Source: CAD feature listing. Evaluate the final solid. Frame: model axes, mm. Face numbers are marked on the shaded views. Coordinates: 2 decimals unless noted, no trailing zeros. Loops run counter-clockwise (first coordinate to the right, second up) from the corner with the lowest first, then second, coordinate; pieces in that order, holes last.
Item 1: Section query D-D, the plane z = -0.45. Return the cut outline in (x, y), then the cut area to 3 significant figures.
Item 2: Section query A-A, the plane x = 0. Return the cut outline in (y, z).
Item 3: Pin query (flat end, axial travel): pin 1 Ø6 at (x, y) = (2, -3.5) entering from +Z; pin 2 Ø5 at (x, y) = (0, 0) entering from -Z; pin 3 Ø1 at (y, z) = (-7.5, -0.5) entering from +X; pin 4 Ø2 at (x, z) = (7.5, 0.5) entering from -Y. Return the tip coordinate at first contact, or that it passes through.
Item 4: Section query C-C, the plane y = -5.5. Return the cut outline in (x, z).
Item 5: Pull-direction query (Y, two-part tool) for the marked faces 1, 2 and 3; classes: +Y half, -Y half, draft (parallel to the pull), parting line (faces both ways), or undercut.
Item 6: Line query: probe 1 along Y at (x, z) = (0, -0.45); probe 2 along Y at (x, z) = (0, 2.9); probe 3 along Z at (x, y) = (-6.25, 1.75). Output: solid intervals per line, ascending.
Autodesk Fusion 360 part; units mm, degrees
sketch "Skizze1" plane through (0, 0, 0) normal (0, 0, 1) x (1, 0, 0)
  line L0 (-39.8802, 0) -> (43.6662, 0) construction
  line L1 (0, 41.7732) -> (0, -47.5785) construction
  circle A0 centre (0, 0) radius 11
  circle A1 centre (0, 0) radius 10.1
  circle A2 centre (0, 0) radius 1.25
  circle A3 centre (0, 0) radius 2.25
  dimension "d1" = 22
  dimension "d2" = 20.2
  dimension "d3" = 2.5
  dimension "d4" = 4.5
extrude "Extrusion1" add sketch "Skizze1" against normal blind 1.5 contours A1 | A3
extrude "Extrusion2" add sketch "Skizze1" along normal blind 1.5 contours A1
extrude "Extrusion3" add sketch "Skizze1" along normal blind 3.5 and the other way blind 1.5 contours A0
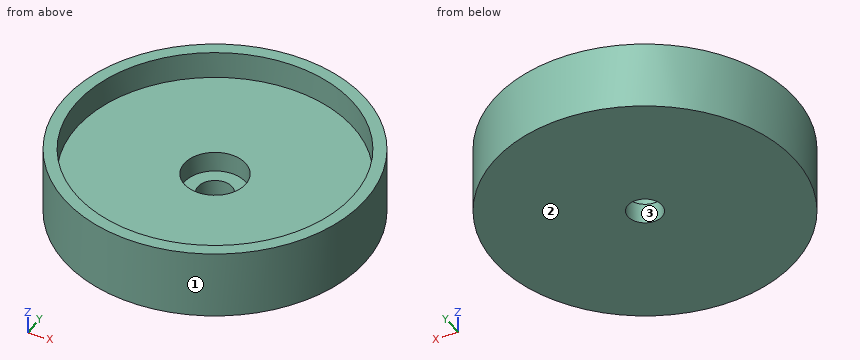
Verdict:
1. outline: circle Ø22 at (0, 0); hole circle Ø2.5 at (0, 0)
1. area: 375 mm2
2. outline: (-11, -1.5) - (-1.25, -1.5) - (-1.25, 0) - (-2.25, 0) - (-2.25, 1.5) - (-10.1, 1.5) - (-10.1, 3.5) - (-11, 3.5) - close; (1.25, -1.5) - (11, -1.5) - (11, 3.5) - (10.1, 3.5) - (10.1, 1.5) - (2.25, 1.5) - (2.25, 0) - (1.25, 0) - close
3. pin 1: stops at z = 1.5
3. pin 2: stops at z = -1.5
3. pin 3: stops at x = 8.49
3. pin 4: stops at y = -8.87
4. outline: (-9.53, -1.5) - (9.53, -1.5) - (9.53, 3.5) - (8.47, 3.5) - (8.47, 1.5) - (-8.47, 1.5) - (-8.47, 3.5) - (-9.53, 3.5) - close
5. face 1: parting line
5. face 2: draft
5. face 3: undercut
6. probe 1: y = -11 to -1.25, 1.25 to 11
6. probe 2: y = -11 to -10.1, 10.1 to 11
6. probe 3: z = -1.5 to 1.5
